Study the drawing (mm; zero at the part's minimum x, y, z) and answer. A direction names the side the tool comes from. Coordinates: 2 decimals unless noted, no trailing zeros. Order: outer loops, then holes, each group sorted by start corner. A loop starts at its lowest first (then second) coordinate and runs counter-clockwise, first axis right, second up.
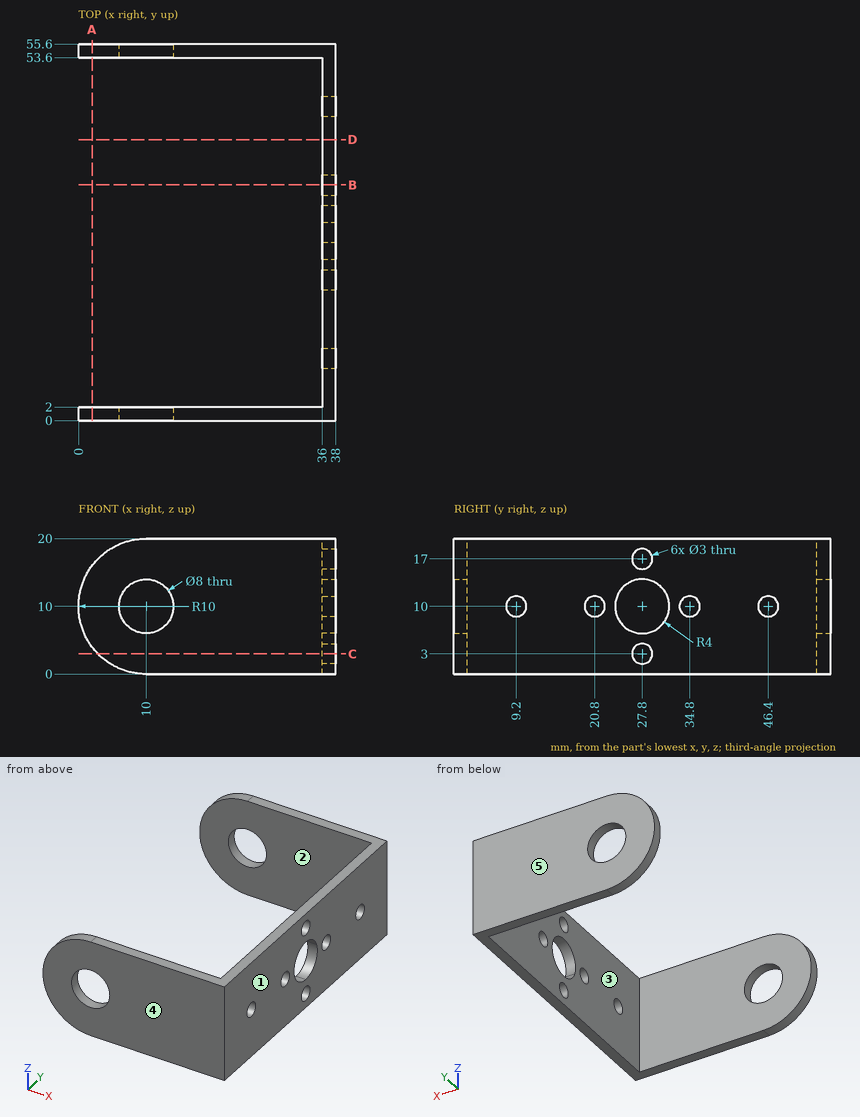
(1) Consider line 1 (Y direction, x = 37.5, z = 10); line 2 (Z direction, x = 37, y = 27); line 3 (Y direction, x = 27, z = 2.75). Determine where each line is inside the solid, lowest interval first.
(2) The mould has two halves that part along Y. Classify the marked faces 3, 4 and 5: released by +Y, released by -Y, zero draft, split by the parting line, or undercut.
(3) This flat-tipped pin is pushed along its axis until it touches: pin 1 Ø4 at (y, z) = (15, 12.5) entering from -X. Where does it stop, or does it pass through?
(4) Find section C-C (z = 3). Write down the section's boundary in (x, y).
(5) Find section B-B (y = 34.8). Write down the section's boundary in (x, z).
(6) For the marked faces 1 and 2, determine the directions among +Z, -Z, +X, -X, +Y, -Y from which every point of the face is accessible in a straight line to the end or side of a thin tool.
(7) Find section D-D (y = 41.5). Write down the section's boundary in (x, z).
(8) Find section A-A (x = 2). Write down the section's boundary in (y, z).
Findings below:
1. line 1: y = 0 to 7.7, 10.7 to 19.3, 22.3 to 23.8, 31.8 to 33.3, 36.3 to 44.9, 47.9 to 55.6
1. line 2: z = 0 to 1.73, 4.27 to 6.08, 13.92 to 15.73, 18.27 to 20
1. line 3: y = 0 to 2, 53.6 to 55.6
2. face 3: undercut
2. face 4: released by -Y
2. face 5: released by +Y
3. pin 1: stops at x = 36
4. outline: (2.86, 0) - (38, 0) - (38, 26.3) - (36, 26.3) - (36, 2) - (2.86, 2) - close; (2.86, 53.6) - (36, 53.6) - (36, 29.3) - (38, 29.3) - (38, 55.6) - (2.86, 55.6) - close
5. outline: (36, 0) - (38, 0) - (38, 8.5) - (36, 8.5) - close; (36, 11.5) - (38, 11.5) - (38, 20) - (36, 20) - close
6. face 1: +Z, -Z, +X, +Y, -Y
6. face 2: +Z, -Z, -X
7. outline: (36, 0) - (38, 0) - (38, 20) - (36, 20) - close
8. outline: (0, 4) - (2, 4) - (2, 16) - (0, 16) - close; (53.6, 4) - (55.6, 4) - (55.6, 16) - (53.6, 16) - close
